The listing builds one solid part. Answer for the finished solid, in the listing's coordinates (mm). A direction names the side the tool comes from. Coordinates: 2 decimals unless noted, no trailing zeros. Loops run counter-clockwise (first coordinate to the right, second up) from the corner with the lowest first, then second, coordinate; pieces in that order, holes last. Notation, with made-up numbers: (84.5, -4) - (115.5, -4) arc R37 cw to (115.5, 32) - close; hole circle Ø7 at (84, 24.25). An arc over 180 degrees is marked (long way). One line per question, with ' | ' between items.
Autodesk Inventor part; units mm, degrees
ref_plane "YZ Plane" through (0, 0, 0) normal (1, 0, 0) x (0, 1, 0)
ref_plane "XZ Plane" through (0, 0, 0) normal (0, 1, 0) x (-1, 0, 0)
ref_plane "XY Plane" through (0, 0, 0) normal (0, 0, 1) x (1, 0, 0)
sketch "Sketch1" plane through (0, 0, 0) normal (0, 1, 0) x (-1, 0, 0)
  line L0 (0, 0) -> (2, 0)
  line L1 (2, 0) -> (2, -4)
  line L2 (2, -4) -> (2.5, -4)
  line L3 (2.5, -4) -> (2.5, -15)
  line L4 (2.5, -15) -> (3.5, -15)
  line L5 (3.5, -15) -> (3.5, -18)
  line L6 (3.5, -18) -> (0, -18)
  line L7 (0, -18) -> (0, 0)
  dimension "d0" = 3
  dimension "d1" = 11
  dimension "d2" = 4
  dimension "d3" = 7
  dimension "d4" = 5
  dimension "d5" = 4
revolve "Revolution1" add sketch "Sketch1" angle 360 about axis through (0, 0, -18) along (0, 0, 1)
thread "Thread1"
properties part number "2053"
Item 1: Find section D-D, the plane z = -16.5. Write down the section's boundary in (x, y).
Taken from the geometry:
outline: circle Ø7 at (0, 0)
Item 2: Which of the six approach directions +Z, -Z, +X, -X, +Y, -Y give full straight-line access (tool end or side, diameter ignored) to faces 1 (the face through (0, 0, 0)), 2 (the face through (1, -2, -4))?
Taken from the geometry:
face 1: +Z, +X, -X, +Y, -Y | face 2: +Z
Item 3: Find section A-A, the plane y = 0. Write down the section's boundary in (x, z), plus the area to 3 significant figures.
Taken from the geometry:
outline: (-3.5, -18) - (3.5, -18) - (3.5, -15) - (2.5, -15) - (2.5, -4) - (2, -4) - (2, 0) - (-2, 0) - (-2, -4) - (-2.5, -4) - (-2.5, -15) - (-3.5, -15) - close | area: 92.0 mm2
Item 4: Find the intervals of material crossed by line 1 (X direction, y = 1.5, z = -7); line 2 (Z direction, x = 3, y = -1.5); line 3 (Z direction, x = -1, y = 2), in increasing order. Write a range as [from, to].
Taken from the geometry:
line 1: x = [-2, 2] | line 2: z = [-18, -15] | line 3: z = [-18, -4]
Item 5: Each of these flat-tipped pins is pushed along its axis until it touches: pin 1 Ø3 at (x, z) = (1.5, -4) entering from +Y; pin 2 Ø1 at (y, z) = (2.5, -7.5) entering from +X. Where does it stop, or does it pass through?
Taken from the geometry:
pin 1: stops at y = 2.5 | pin 2: stops at x = 1.5
Item 6: Find section C-C, the plane z = -2.5. Write down the section's boundary in (x, y), plus the area to 3 significant figures.
Taken from the geometry:
outline: circle Ø4 at (0, 0) | area: 12.6 mm2
